Geometry check sheet. Reference: the model listing, model coordinates, mm. A direction names the side the tool comes from. Coordinates: 2 decimals unless noted, no trailing zeros. Order: outer loops, then holes, each group sorted by start corner. A loop starts at its lowest first (then second) coordinate and runs counter-clockwise, first axis right, second up. Notation, with made-up numbers: (79.25, -38) - (97.25, -38) arc R19 cw to (97.25, -31) - close; hole circle Ø11 at (17, -36). An arc over 180 degrees is marked (long way). Use CSV: the item, a comma, the result in double quotes. Start each with the question number.
1) Tool access check on faces 4 (the flat face through (12.4, 6.275, 0.2)), 5 (the flat face through (1.09, 5.5, -1.5)), 6 (the flat face through (17, -2, 0.55)), 7 (the flat face through (-2, 5, -2.54)). Record the directions out of +Z, -Z, +X, -X, +Y, -Y that give a thin tool (end or side, any length) a straight path to the whole face; none if there is none.
2) Sectioned sample at A-A, the plane z = -4. Record the cut outline in (x, y) (3 decimals), and give its area (3 significant figures).
3) Sectioned sample at C-C, the plane z = 5.25. Count the separate pieces of the cut face and the enclosed holes in it, and give its area (3 significant figures).
4) Sectioned sample at D-D, the plane x = 11.08. Record the cut outline in (y, z) (3 decimals).
5) Draft check along X on faces 1 (the cylindrical face through (12.32, -1.56, 3.44)), 2 (the flat face through (-2.91, -4, -4)), 3 (the flat face through (26.2, 1.1, -4.38)). Enter one of: released by +X, released by -X, zero draft, split by the parting line, or undercut.
6) Depth check by flat-ended pin: P1, Ø10, axis at x = 17, z = -8.5, coming from the +Y side (3 decimals); P2, Ø3, axis at y = 1.5, z = 4, coming from the +X side; P3, Ø1.1, axis at x = 1, z = -3, coming from the +Y side (3 decimals). Enter the tip coordinate at first touch or a pass-through.
7) Sectioned sample at B-B, the plane x = 24.99. Record the cut outline in (y, z) (3 decimals), and give its area (3 significant figures).
8) Thickness scan on probe 1 along Y at (x, z) = (16.8, 2.55); probe 2 along X at (y, z) = (0, -2.1); probe 3 along Z at (x, y) = (14, 3). Record the ranges inside material, lowest first. Write a range as [from, to].
from build123d import *
from build123d.topology import SkipClean

# Parameters (mm, degrees)
SKETCH1_R                 = 1.58
BASE_EXTRUDE_DEPTH        = 0.43
ENGAGEMENT_D_DEPTH        = 6.17
ENGAGEMENT_RADII_R        = 0.5
TOP_START                 = -2.54
TOP_CUT_OUT_OUTLINE_W     = 30.81
TOP_CUT_OUT_OUTLINE_H     = 2.76
TOP_CUT_OUT_DEPTH         = 14.5
TOP_CUT_OUT_2_OUTLINE_W   = 30.81
TOP_CUT_OUT_2_OUTLINE_H   = 6.65
TOP_CUT_OUT_2_DEPTH       = 3.47
TOP_CUT_OUT_3_OUTLINE_W   = 1.31
TOP_CUT_OUT_3_OUTLINE_H   = 2.99
TOP_CUT_OUT_3_OUTLINE_W_2 = 21.79
TOP_CUT_OUT_3_DEPTH       = 2.54
TOP_CUT_OUT_4_OUTLINE_W   = 3.2
TOP_CUT_OUT_4_OUTLINE_H   = 2.99
TOP_CUT_OUT_4_DEPTH       = 1.34
TAB_TOP_DEPTH             = 1.09
SKETCH15_R                = 1.45
NUT_DEPTH                 = 0.91
NUT_HOLE_REACH            = 32.65
SKETCH16_R                = 1.45
CUT_EXTRUDE9_DEPTH        = 0.05
SKETCH20_W                = 16.32
SKETCH20_H                = 11.96
BOSS_EXTRUDE1_DEPTH       = 9.64
SKETCH25_W                = 0.43
SKETCH25_H                = 11.55
CUT_EXTRUDE13_DEPTH       = 0.1
SKETCH26_W                = 0.43
SKETCH26_H                = 11.55
CUT_EXTRUDE14_DEPTH       = 0.1
SKETCH30_R                = 0.45
CUT_EXTRUDE16_DEPTH       = 6
LPATTERN1_COUNT           = 5
LPATTERN1_PITCH           = 2.29
CHAMFER1_SIZE             = 0.3


# Read off the part's stored shape, not the designer's step: top cut out
with BuildPart() as part:
    # Sketch1 → Base-Extrude (new body)
    with BuildSketch(Plane.XY):
        Polygon((-2.91, 6.275), (27.9, 6.275), (27.9, -5.275), (22.9, -5.275), (22.322649731, -6.275), (2.667350269, -6.275), (2.09, -5.275), (-2.91, -5.275), align=None)
        Circle(SKETCH1_R, mode=Mode.SUBTRACT)
        with Locations((24.99, 0)):
            Circle(SKETCH1_R, mode=Mode.SUBTRACT)
    extrude(amount=BASE_EXTRUDE_DEPTH)

    # Sketch2 → engagement D (add)
    with BuildSketch(Plane.XY.offset(0.43)):
        with BuildLine():
            Line((6.3, 4), (18.69, 4))
            ThreePointArc((18.69, 4), (20.222088886, 3.285575219), (20.659615506, 1.652703645))
            Line((20.659615506, 1.652703645), (19.954307583, -2.347296355))
            ThreePointArc((19.954307583, -2.347296355), (19.270267297, -3.532088886), (17.984692077, -4))
            Line((17.984692077, -4), (7.005307923, -4))
            ThreePointArc((7.005307923, -4), (5.719732703, -3.532088886), (5.035692417, -2.347296355))
            Line((5.035692417, -2.347296355), (4.330384494, 1.652703645))
            ThreePointArc((4.330384494, 1.652703645), (4.767911114, 3.285575219), (6.3, 4))
        make_face()
    extrude(amount=ENGAGEMENT_D_DEPTH)

    # engagement radii
    engagement_radii_edges = [part.edges().sort_by_distance(p)[0] for p in [
        (20.222088886, 3.285575219, 0.43),
        (12.495, 4, 6.6),
        (4.767911114, 3.285575219, 6.6),
        (4.683038455, -0.347296355, 0.43),
        (5.719732703, -3.532088886, 6.6),
        (12.495, -4, 0.43),
        (19.270267297, -3.532088886, 0.43),
        (20.306961545, -0.347296355, 6.6),
        (20.222088886, 3.285575219, 6.6),
        (4.683038455, -0.347296355, 6.6),
        (12.495, -4, 6.6),
        (19.270267297, -3.532088886, 6.6),
        (20.306961545, -0.347296355, 0.43),
        (5.719732703, -3.532088886, 0.43),
        (4.767911114, 3.285575219, 0.43),
        (12.495, 4, 0.43),
    ]]
    fillet(engagement_radii_edges, radius=ENGAGEMENT_RADII_R)

    # top cut out outline → top cut out (add)
    with BuildSketch(Plane(origin=(0, 0, -2.54), x_dir=(-1, 0, 0), z_dir=(0, 0, -1)).offset(TOP_START)):
        with Locations((-12.495, -4.895)):
            Rectangle(TOP_CUT_OUT_OUTLINE_W, TOP_CUT_OUT_OUTLINE_H)
    extrude(amount=TOP_CUT_OUT_DEPTH)

    # top cut out 2 outline → top cut out 2 (add)
    with BuildSketch(Plane(origin=(0, 0, -2.54), x_dir=(-1, 0, 0), z_dir=(0, 0, -1)).offset(TOP_START)):
        with Locations((-12.495, -0.19)):
            Rectangle(TOP_CUT_OUT_2_OUTLINE_W, TOP_CUT_OUT_2_OUTLINE_H)
    extrude(amount=TOP_CUT_OUT_2_DEPTH)

    # top cut out 3 outline → top cut out 3 (add)
    with BuildSketch(Plane(origin=(0, 0, -2.54), x_dir=(-1, 0, 0), z_dir=(0, 0, -1)).offset(TOP_START)):
        with Locations((-27.245, 4.63)):
            Rectangle(TOP_CUT_OUT_3_OUTLINE_W, TOP_CUT_OUT_3_OUTLINE_H)
        with Locations((-12.495, 4.63)):
            Rectangle(TOP_CUT_OUT_3_OUTLINE_W_2, TOP_CUT_OUT_3_OUTLINE_H)
        with Locations((2.255, 4.63)):
            Rectangle(TOP_CUT_OUT_3_OUTLINE_W, TOP_CUT_OUT_3_OUTLINE_H)
    extrude(amount=TOP_CUT_OUT_3_DEPTH)

    # top cut out 4 outline → top cut out 4 (add)
    with BuildSketch(Plane(origin=(0, 0, -2.54), x_dir=(-1, 0, 0), z_dir=(0, 0, -1)).offset(TOP_START)):
        with Locations((-24.99, 4.63)):
            Rectangle(TOP_CUT_OUT_4_OUTLINE_W, TOP_CUT_OUT_4_OUTLINE_H)
        with Locations((0, 4.63)):
            Rectangle(TOP_CUT_OUT_4_OUTLINE_W, TOP_CUT_OUT_4_OUTLINE_H)
    extrude(amount=TOP_CUT_OUT_4_DEPTH)

    # Sketch14 → tab top (add, symmetric)
    with BuildSketch(Plane(origin=(0, 0, 0), x_dir=(0, 0, -1), z_dir=(1, 0, 0))):
        with BuildLine():
            Line((1.34, 5.725), (1.34, 4.335))
            Line((1.34, 4.335), (1.79, 4.335))
            Line((1.79, 4.335), (1.79, 5.725))
            ThreePointArc((1.79, 5.725), (1.62890873, 6.11390873), (1.24, 6.275))
            Line((1.24, 6.275), (0, 6.275))
            Line((0, 6.275), (0, 5.825))
            Line((0, 5.825), (1.24, 5.825))
            ThreePointArc((1.24, 5.825), (1.310710678, 5.795710678), (1.34, 5.725))
        make_face()
    tab_top = extrude(amount=TAB_TOP_DEPTH, both=True)

    # tab 2: tab top across plane
    add(tab_top.mirror(Plane(origin=(12.495, 0, 0), x_dir=(0, 0, 1), z_dir=(1, 0, 0))))

    # Sketch15 → nut (add)
    with BuildSketch(Plane(origin=(0, 0, -3.47), x_dir=(-1, 0, 0), z_dir=(0, 0, -1))):
        Polygon((2.886751346, 0), (1.443375673, 2.5), (-1.443375673, 2.5), (-2.886751346, 0), (-1.443375673, -2.5), (1.443375673, -2.5), align=None)
        with Locations(Location((0, 0, 0), (0, 0, 90))):
            Circle(SKETCH15_R, mode=Mode.SUBTRACT)
    nut = extrude(amount=NUT_DEPTH)

    # Sketch16 → nut hole (cut, up to next)
    with BuildSketch(Plane(origin=(0, 0, -3.47), x_dir=(-1, 0, 0), z_dir=(0, 0, -1)), mode=Mode.PRIVATE) as nut_hole_sk1:
        Circle(SKETCH16_R)
    nut_hole_tool1 = extrude(nut_hole_sk1.sketch, amount=-NUT_HOLE_REACH, mode=Mode.PRIVATE) & part.part
    nut_hole = nut_hole_tool1.solids().sort_by_distance((0, 0, -3.47))[0]
    add(nut_hole, mode=Mode.SUBTRACT)

    # nut 2: nut, nut hole across plane
    with SkipClean():  # the faces are left unmerged after this step: merging them gives an invalid solid
        add(nut.mirror(Plane(origin=(12.495, 0, 0), x_dir=(0, 0, 1), z_dir=(1, 0, 0))))
        add(nut_hole.mirror(Plane(origin=(12.495, 0, 0), x_dir=(0, 0, 1), z_dir=(1, 0, 0))), mode=Mode.SUBTRACT)

    # Sketch18 → Cut-Extrude9 (cut)
    with SkipClean():  # the faces are left unmerged after this step: merging them gives an invalid solid
        with BuildSketch(Plane.XY.offset(6.6)):
            with BuildLine():
                Line((19.461903707, -2.260472267), (20.16721163, 1.739527733))
                ThreePointArc((20.16721163, 1.739527733), (19.839066665, 2.964181415), (18.69, 3.5))
                Line((18.69, 3.5), (6.3, 3.5))
                ThreePointArc((6.3, 3.5), (5.150933335, 2.964181415), (4.82278837, 1.739527733))
                Line((4.82278837, 1.739527733), (5.528096293, -2.260472267))
                ThreePointArc((5.528096293, -2.260472267), (6.041126508, -3.149066665), (7.005307923, -3.5))
                Line((7.005307923, -3.5), (17.984692077, -3.5))
                ThreePointArc((17.984692077, -3.5), (18.948873492, -3.149066665), (19.461903707, -2.260472267))
            make_face()
        extrude(amount=-CUT_EXTRUDE9_DEPTH, mode=Mode.SUBTRACT)

    # Sketch20 → Boss-Extrude1 (add)
    with SkipClean():  # the faces are left unmerged after this step: merging them gives an invalid solid
        with BuildSketch(Plane(origin=(0, -3.515, 0), x_dir=(-1, 0, 0), z_dir=(0, 1, 0))):
            with Locations((-12.495, -8.52)):
                Rectangle(SKETCH20_W, SKETCH20_H)
        extrude(amount=BOSS_EXTRUDE1_DEPTH)

    # Sketch25 → Cut-Extrude13 (cut)
    with SkipClean():  # the faces are left unmerged after this step: merging them gives an invalid solid
        with BuildSketch(Plane(origin=(27.9, 0, 0), x_dir=(0, 0, -1), z_dir=(1, 0, 0))):
            with Locations((-0.215, 0.5)):
                Rectangle(SKETCH25_W, SKETCH25_H)
        extrude(amount=-CUT_EXTRUDE13_DEPTH, mode=Mode.SUBTRACT)

    # Sketch26 → Cut-Extrude14 (cut)
    with SkipClean():  # the faces are left unmerged after this step: merging them gives an invalid solid
        with BuildSketch(Plane.ZY.offset(2.91)):
            with Locations((0.215, 0.5)):
                Rectangle(SKETCH26_W, SKETCH26_H)
        extrude(amount=-CUT_EXTRUDE14_DEPTH, mode=Mode.SUBTRACT)

    # Sketch30 → Cut-Extrude16 (cut)
    with SkipClean():  # the faces are left unmerged after this step: merging them gives an invalid solid
        with BuildSketch(Plane.XY.offset(6.55)):
            with Locations((16.8, 2)):
                Circle(SKETCH30_R)
            with Locations(Location((16.8, -2, 0), (0, 0, 180))):
                Circle(SKETCH30_R)
            with Locations((17.95, 0)):
                Circle(SKETCH30_R)
        cut_extrude16 = extrude(amount=-CUT_EXTRUDE16_DEPTH, mode=Mode.SUBTRACT)

    # LPattern1: Cut-Extrude16 ×5
    with SkipClean():  # the faces are left unmerged after this step: merging them gives an invalid solid
        with Locations(*[(-i * LPATTERN1_PITCH, 0, 0) for i in range(1, LPATTERN1_COUNT)]):
            add(cut_extrude16, mode=Mode.SUBTRACT)

    # Chamfer1
    chamfer1_edges = [part.edges().sort_by_distance(p)[0] for p in [
        (16.35, 2, 6.55),
        (17.25, -2, 6.55),
        (17.5, 0, 6.55),
        (14.06, 2, 6.55),
        (14.96, -2, 6.55),
        (15.21, 0, 6.55),
        (11.77, 2, 6.55),
        (12.67, -2, 6.55),
        (12.92, 0, 6.55),
        (9.48, 2, 6.55),
        (10.38, -2, 6.55),
        (10.63, 0, 6.55),
        (7.19, 2, 6.55),
        (8.09, -2, 6.55),
        (8.34, 0, 6.55),
    ]]
    chamfer(chamfer1_edges, length=CHAMFER1_SIZE)


solid = part.part
Evaluation:
1,face 4,"+Z, -Z, +X, -X, +Y"
1,face 5,"-Z, +Y"
1,face 6,"+Z"
1,face 7,"-Z, -X, +Y"
2,outline,"(-2.91, -6.275) - (27.9, -6.275) - (27.9, -3.515) - (20.655, -3.515) - (20.655, 6.125) - (4.335, 6.125) - (4.335, -3.515) - (-2.91, -3.515) - close; (-2.887, 0) - (-1.443, -2.5) - (1.443, -2.5) - (2.887, 0) - (1.443, 2.5) - (-1.443, 2.5) - close; (22.103, 0) - (23.547, -2.5) - (26.433, -2.5) - (27.877, 0) - (26.433, 2.5) - (23.547, 2.5) - close; hole circle Ø2.9 at (0, 0); hole circle Ø2.9 at (24.99, 0)"
2,area,"272 mm²"
3,separate pieces,"1"
3,enclosed holes,"15"
3,area,"113 mm²"
4,outline,"(-6.275, -14.5) - (6.125, -14.5) - (6.125, 0) - (6.275, 0) - (6.275, 0.43) - (4.5, 0.43) arc R0.5 cw to (4, 0.93) - (4, 6.1) arc R0.5 ccw to (3.5, 6.6) - (3.5, 6.55) - (0.75, 6.55) - (0.45, 6.25) - (0.45, 0.55) - (-0.45, 0.55) - (-0.45, 6.25) - (-0.75, 6.55) - (-3.5, 6.55) - (-3.5, 6.6) arc R0.5 ccw to (-4, 6.1) - (-4, 0.93) arc R0.5 cw to (-4.5, 0.43) - (-6.275, 0.43) - close"
5,face 1,"undercut"
5,face 2,"released by -X"
5,face 3,"zero draft"
6,P1,"y = 6.125"
6,P2,"x = 20.69"
6,P3,"y = 3.135"
7,outline,"(-6.275, -14.5) - (-3.515, -14.5) - (-3.515, -3.47) - (-2.5, -3.47) - (-2.5, -4.38) - (-1.45, -4.38) - (-1.45, 0) - (-1.58, 0) - (-1.58, 0.43) - (-5.275, 0.43) - (-5.275, 0) - (-6.275, 0) - close; (1.45, -4.38) - (2.5, -4.38) - (2.5, -3.47) - (3.135, -3.47) - (3.135, -1.34) - (4.335, -1.34) - (4.335, -1.79) - (5.725, -1.79) arc R0.55 ccw to (6.275, -1.24) - (6.275, 0.43) - (1.58, 0.43) - (1.58, 0) - (1.45, 0) - close"
7,area,"63.6 mm²"
8,probe 1,"[-4, -2.45], [-1.55, 1.55], [2.45, 4]"
8,probe 2,"[-2.91, -1.45], [1.45, 23.54], [26.44, 27.9]"
8,probe 3,"[-14.5, 6.55]"
